Study the drawing (mm; zero at the part's minimum x, y, z) and answer. A direction names the side the tool comes from. Round coordinates to 2 decimals unless told otherwise and drop trailing zeros. Write each loop counter-clockwise with the first axis right and the second up, starting at its lowest first coordinate (ties: lowest second). Pieces come first, ordered by that corner, then holes. Notation, with made-up numbers: (49.25, 21) -> (81.25, 21) arc R25 cw to (81.25, 39) -> close; hole circle Ø5 at (73.5, -9). An arc over 180 degrees is marked (long way). Return JSON: item names as keys, results as strings.
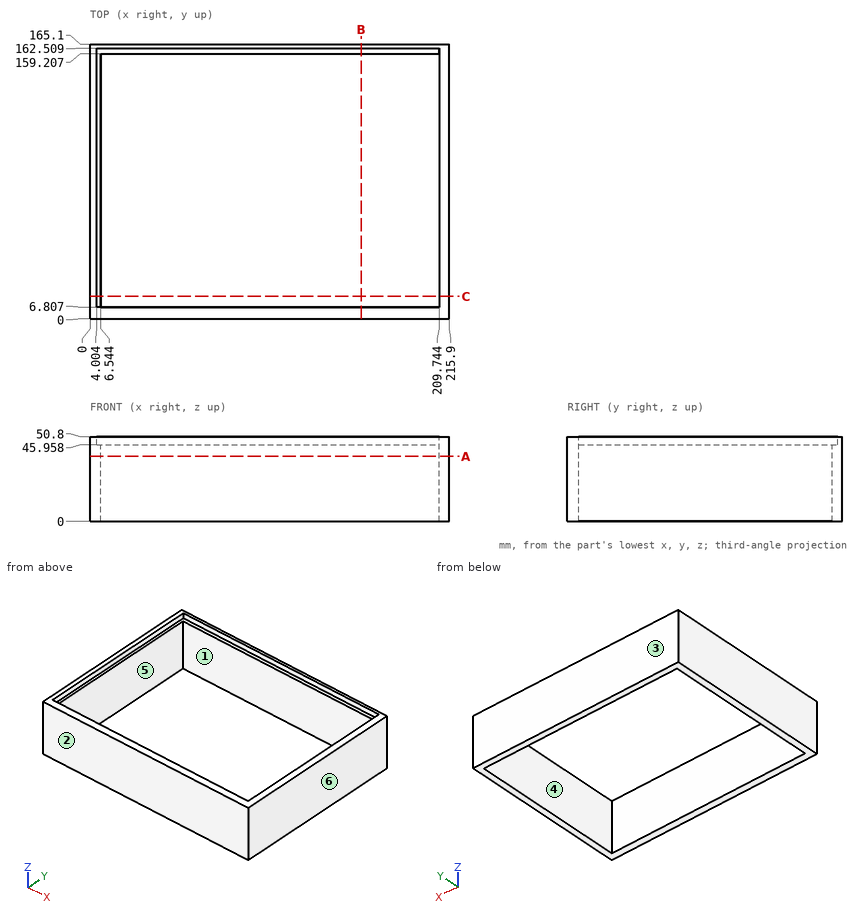
Item 1: For a pull along Y with two mould halves and no side action, classify the marked faces 3, 4, 5 and 6 as released by +Y, released by -Y, zero draft, split by the parting line, or undercut.
Worked answers:
{"face 3": "released by +Y", "face 4": "undercut", "face 5": "undercut", "face 6": "zero draft"}
Item 2: Section C-C (y = 13.5) is taken. Give the vertices of the cut face in (x, z), then the cut area to 3 significant figures.
Worked answers:
{"outline": "(0, 0) -> (6.54, 0) -> (6.54, 45.96) -> (4, 45.96) -> (4, 50.8) -> (0, 50.8) -> close; (209.74, 0) -> (215.9, 0) -> (215.9, 50.8) -> (209.74, 50.8) -> close", "area": "633 mm2"}
Item 3: Section A-A (z = 39) is taken. Give the vertices of the cut face in (x, y).
Worked answers:
{"outline": "(0, 0) -> (215.9, 0) -> (215.9, 165.1) -> (0, 165.1) -> close; hole (6.54, 6.81) -> (209.74, 6.81) -> (209.74, 159.21) -> (6.54, 159.21) -> close"}
Item 4: Section B-B (x = 163) is taken. Give the vertices of the cut face in (y, z).
Worked answers:
{"outline": "(0, 0) -> (6.81, 0) -> (6.81, 50.8) -> (0, 50.8) -> close; (159.21, 0) -> (165.1, 0) -> (165.1, 50.8) -> (162.51, 50.8) -> (162.51, 45.96) -> (159.21, 45.96) -> close"}
Item 5: Straight lines are drawn through the part: L1, parallel to Y at x = 126, z = 24; L2, parallel to X at y = 138.5, z = 36.5; L3, parallel to X at y = 84.5, z = 48. For each, find the intervals that lie inside material, in ascending order. Write a range as [from, to].
Worked answers:
{"L1": "y = [0, 6.81], [159.21, 165.1]", "L2": "x = [0, 6.54], [209.74, 215.9]", "L3": "x = [0, 4], [209.74, 215.9]"}
Item 6: A tool of negligible diameter and unlimited length cuts with its end or side. For the marked faces 1 and 2, from which of +Z, -Z, +X, -X, +Y, -Y can it reach the whole face along a straight path? Write none if from no direction.
Worked answers:
{"face 1": "+Z, -Z", "face 2": "+Z, -Z, +X, -X, -Y"}
